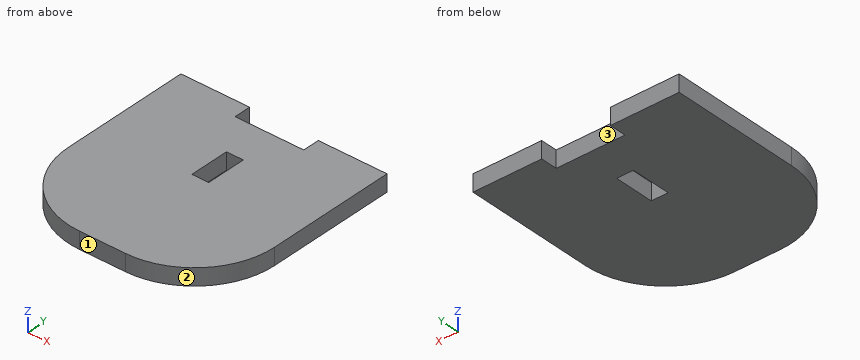
from build123d import *

# Parameters (mm, degrees)
SKETCH1_W           = 65.278
SKETCH1_H           = 66.675
BOSS_EXTRUDE1_DEPTH = 5.334
SKETCH2_W           = 21.759333334
SKETCH2_H           = 5.334
CUT_EXTRUDE1_DEPTH  = 152.591443439
FILLET1_R           = 25.4
FILLET2_R           = 25.4
SKETCH3_W           = 5.334
SKETCH3_H           = 12.7
CUT_EXTRUDE2_DEPTH  = 152.591443439


with BuildPart() as part:
    # Sketch1 → Boss-Extrude1 (new body)
    with BuildSketch(Plane.XY):
        with Locations((-63.136117913, 84.044955915)):
            Rectangle(SKETCH1_W, SKETCH1_H)
    extrude(amount=BOSS_EXTRUDE1_DEPTH)

    # Sketch2 → Cut-Extrude1 (cut, through all)
    with BuildSketch(Plane.XY.offset(5.334)):
        with Locations((-63.136117913, 114.715455915)):
            Rectangle(SKETCH2_W, SKETCH2_H)
    extrude(amount=-CUT_EXTRUDE1_DEPTH, mode=Mode.SUBTRACT)

    # Fillet1
    fillet1_edges = [part.edges().sort_by_distance(p)[0] for p in [
        (-95.775117913, 50.707455915, 2.667),
    ]]
    fillet(fillet1_edges, radius=FILLET1_R)

    # Fillet2
    fillet2_edges = [part.edges().sort_by_distance(p)[0] for p in [
        (-30.497117913, 50.707455915, 2.667),
    ]]
    fillet(fillet2_edges, radius=FILLET2_R)

    # Sketch3 → Cut-Extrude2 (cut, through all)
    with BuildSketch(Plane.XY.offset(5.334)):
        with Locations((-63.136117913, 92.998455915)):
            Rectangle(SKETCH3_W, SKETCH3_H)
    extrude(amount=-CUT_EXTRUDE2_DEPTH, mode=Mode.SUBTRACT)


solid = part.part
Read the model definition and answer for the solid it produces. Units are mm, in the model's axes. Face numbers are marked on the shaded views. Give positions to 0.01 mm unless a question says otherwise; leave off trailing zeros. Write each loop counter-clockwise with the first axis right and the second up, starting at its lowest first coordinate (ties: lowest second). Pieces come first, ordered by that corner, then holes. Notation, with made-up numbers: (4.25, 53.5) -> (10.25, 53.5) arc R30 ccw to (10.25, 91.5) -> close; hole circle Ø11 at (53.5, -19). An arc over 180 degrees is marked (long way). Answer as a JSON object with one key per item and string values. Group by question number.
1) The mould has two halves that part along X. Classify the marked faces 1, 2 and 3: +X half, -X half, draft (parallel to the pull), parting line (faces both ways), or undercut.
2) Find section B-B (z = 3.05). Write down the section's boundary in (x, y).
3) This flat-tipped pin is pushed along its axis until it touches: P1, Ø1.6, axis at x = -62.5, z = 3, coming from the +Y side. Where does it stop, or does it pass through?
4) Find section C-C (x = -62). Write down the section's boundary in (y, z), and give its area (3 significant figures).
5) Find section A-A (y = 92). Write down the section's boundary in (x, z), and give its area (3 significant figures).
6) Find section D-D (x = -77.5). Write down the section's boundary in (y, z).
7) Consider L1, parallel to X at y = 98.5, z = 3.5; L2, parallel to Y at x = -61.5, z = 4.7; L3, parallel to Y at x = -56.5, z = 3.3. Determine where each line is inside the solid, lowest interval first. Write a range as from..to.
Values follow:
{
 "1": {"face 1": "draft", "face 2": "+X half", "face 3": "undercut"},
 "2": {"outline": "(-95.78, 76.11) arc R25.4 ccw to (-70.38, 50.71) -> (-55.9, 50.71) arc R25.4 ccw to (-30.5, 76.11) -> (-30.5, 117.38) -> (-52.26, 117.38) -> (-52.26, 112.05) -> (-74.02, 112.05) -> (-74.02, 117.38) -> (-95.78, 117.38) -> close; hole (-65.8, 86.65) -> (-60.47, 86.65) -> (-60.47, 99.35) -> (-65.8, 99.35) -> close"},
 "3": {"P1": "stops at y = 112.05"},
 "4": {"outline": "(50.71, 0) -> (86.65, 0) -> (86.65, 5.33) -> (50.71, 5.33) -> close; (99.35, 0) -> (112.05, 0) -> (112.05, 5.33) -> (99.35, 5.33) -> close", "area": "259 mm2"},
 "5": {"outline": "(-95.78, 0) -> (-65.8, 0) -> (-65.8, 5.33) -> (-95.78, 5.33) -> close; (-60.47, 0) -> (-30.5, 0) -> (-30.5, 5.33) -> (-60.47, 5.33) -> close", "area": "320 mm2"},
 "6": {"outline": "(51.73, 0) -> (117.38, 0) -> (117.38, 5.33) -> (51.73, 5.33) -> close"},
 "7": {"L1": "x = -95.78..-65.8, -60.47..-30.5", "L2": "y = 50.71..86.65, 99.35..112.05", "L3": "y = 50.71..112.05"}
}
